The model under review builds one solid part; all positions refer to its coordinate system, in mm. A direction names the side the tool comes from. Give positions to 0.01 mm unless a question says otherwise; leave off trailing zeros. Loops run counter-clockwise (first coordinate to the right, second up) from the corner with the lowest first, then second, coordinate; pieces in that order, holes last. Notation, with made-up numbers: M 69.25,37.25 L 128.25,37.25 A16 cw 128.25,60.25 Z; hole C 20,-21 d10. An arc over 180 degrees is marked long. Write item = value, one per line. Start each with the question number.
1. We need section C-C on x = 52. Give the boundary of the cut face in (y, z) (3 decimals), then the cut area to 3 significant figures.
2. For faces 4 (the face through (101.6, -2, 44)), 5 (the face through (0, -52, 44)), 6 (the face through (65, -101.6, 34)), list the 3-axis set-ups (+Z, -Z, +X, -X, +Y, -Y) from which the entire face can be reached by the end or side of a thin tool; tool diameter is ignored.
3. Wall thickness on line 1 along Y through (x, z) = (33.5, 8) (3 decimals); line 2 along X through (y, z) = (-102, 44) (3 decimals); line 3 along X through (y, z) = (-72.5, 53) (3 decimals): over which ranges is each line inside the solid? List them lowest first. Write a range as from..to.
4. For pin 1 (1.5 mm diameter, centred on y = -37, z = 29.5, fed in from +X) (3 decimals); pin 2 (1 mm diameter, centred on y = -1.5, z = 31.5, fed in from +X); pin 3 (12 mm diameter, centred on x = 86, y = -90.5, fed in from +Z), all flat-tipped, find the tip position at first contact; note any pin that passes through.
5. We need section B-B on x = 30. Give the boundary of the cut face in (y, z) (3 decimals), then the cut area to 3 significant figures.
6. We need section D-D on z = 21.5. Give the boundary of the cut face in (x, y) (3 decimals).
7. Draft analysis for pull direction Z (two halves, no side actions). For faces 1 (the face through (2, -53, 0)), 2 (the face through (55.829, -103.21, 59.947)), 3 (the face through (3.175, -52, 44)), state which applies: pulls with the +Z half, pulls with the -Z half, needs draft (parallel to the pull), parting line crosses it, or undercut.
from build123d import *

# Parameters (mm, degrees)
F0_W     = 101.6
F0_H     = 88.9
F1_DEPTH = 3.175
F2_W     = 3.175
F2_H     = 88.9
F3_DEPTH = 101.6
F4_W     = 3.175
F4_H     = 88.9
F5_DEPTH = 101.6
F7_DEPTH = 3.175
F8_R     = 3.175


with BuildPart() as f1:
    # F0 (on Front) → F1 (new body)
    with BuildSketch(Plane.XZ):
        with Locations((50.8, 44.45)):
            Rectangle(F0_W, F0_H)
    extrude(amount=F1_DEPTH)

    # F2 (on face) → F3 (join)
    with BuildSketch(Plane.XZ.offset(3.175)):
        with Locations((1.5875, 44.45)):
            Rectangle(F2_W, F2_H)
    extrude(amount=F3_DEPTH)

    # F4 (on face) → F5 (join)
    with BuildSketch(Plane.YZ.offset(3.175)):
        with Locations((-103.1875, 44.45)):
            Rectangle(F4_W, F4_H)
    extrude(amount=F5_DEPTH)

    # F6 (on face) → F7 (cut, through all)
    with BuildSketch(Plane.XZ.offset(104.775)):
        with BuildLine():
            Line((36.5125, 44.45), (68.2625, 44.45))
            ThreePointArc((68.2625, 44.45), (52.3875, 60.325), (36.5125, 44.45))
        make_face()
        with BuildLine():
            ThreePointArc((36.5125, 44.45), (52.3875, 28.575), (68.2625, 44.45))
            Line((68.2625, 44.45), (36.5125, 44.45))
        make_face()
    extrude(amount=-F7_DEPTH, mode=Mode.SUBTRACT)

    # F8
    f8_edges = [f1.edges().sort_by_distance(p)[0] for p in [
        (0, -104.775, 44.45),
        (0, 0, 44.45),
    ]]
    fillet(f8_edges, radius=F8_R)


solid = f1.part
Final values:
q1.outline = M -104.775,0 L -101.6,0 L -101.6,28.58 L -104.775,28.58 Z; M -104.775,60.32 L -101.6,60.32 L -101.6,88.9 L -104.775,88.9 Z; M -3.175,0 L 0,0 L 0,88.9 L -3.175,88.9 Z
q1.area = 464 mm²
q2.face_4 = +Z, -Z, +X, +Y
q2.face_5 = +Z, -Z, -X, +Y, -Y
q2.face_6 = +Z, -Z, +X
q3.line_1 = -104.775..-101.6, -3.175..0
q3.line_2 = 0.025..36.519, 68.256..104.775
q3.line_3 = 0..3.175
q4.pin_1 = 3.175
q4.pin_2 = 101.6
q4.pin_3 = through
q5.outline = M -104.775,0 L -101.6,0 L -101.6,88.9 L -104.775,88.9 Z; M -3.175,0 L 0,0 L 0,88.9 L -3.175,88.9 Z
q5.area = 565 mm²
q6.outline = M 0,-101.6 A3.175 ccw 3.175,-104.775 L 104.775,-104.775 L 104.775,-101.6 L 3.175,-101.6 L 3.175,-3.175 L 101.6,-3.175 L 101.6,0 L 3.175,0 A3.175 ccw 0,-3.175 Z
q7.face_1 = pulls with the -Z half
q7.face_2 = undercut
q7.face_3 = needs draft
